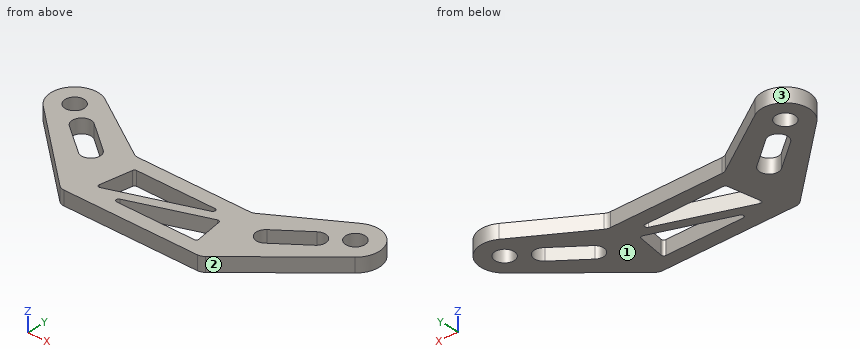
from build123d import *

# Parameters (mm, degrees)
SKETCH_1_R          = 2.025
EXTRUDE_1_DEPTH     = 3
CUT_EXTRUDE_1_DEPTH = 13
FILLET_1_R          = 0.5
FILLET_2_R          = 2


with BuildPart() as part:
    # 草图1 → 凸台-拉伸1 (new body)
    with BuildSketch(Plane.XY):
        with BuildLine():
            Line((-12.5, -5), (-27.339189471, 4.262711851))
            ThreePointArc((-27.339189471, 4.262711851), (-34.026108353, 3.006838294), (-33.33194179, -3.761487592))
            Line((-33.33194179, -3.761487592), (-15, -20))
            Line((-15, -20), (15, -20))
            Line((15, -20), (33.33194179, -3.761487592))
            ThreePointArc((33.33194179, -3.761487592), (34.026108353, 3.006838294), (27.339189471, 4.262711851))
            Line((27.339189471, 4.262711851), (12.5, -5))
            Line((12.5, -5), (-12.5, -5))
        make_face()
        with Locations((-30, 0)):
            Circle(SKETCH_1_R, mode=Mode.SUBTRACT)
        with Locations((30, 0)):
            Circle(SKETCH_1_R, mode=Mode.SUBTRACT)
    extrude(amount=EXTRUDE_1_DEPTH)

    # 草图2 → 切除-拉伸1 (cut)
    with BuildSketch(Plane.XY.offset(3)):
        Polygon((9.958618735, -8), (-9.958618735, -8), (-11.278048465, -15.916578379), align=None)
        Polygon((10.293550357, -10.009589734), (-8.458618735, -17), (11.458618735, -17), align=None)
        with BuildLine():
            Line((17.485082522, -7.103595065), (23.826074435, -2.225908978))
            ThreePointArc((23.826074435, -2.225908978), (26.630743935, -2.591735435), (26.264917478, -5.396404935))
            Line((26.264917478, -5.396404935), (19.923925565, -10.274091022))
            ThreePointArc((19.923925565, -10.274091022), (17.119256065, -9.908264565), (17.485082522, -7.103595065))
        make_face()
        with BuildLine():
            Line((-23.826074435, -2.225908978), (-17.485082522, -7.103595065))
            ThreePointArc((-17.485082522, -7.103595065), (-17.119256065, -9.908264565), (-19.923925565, -10.274091022))
            Line((-19.923925565, -10.274091022), (-26.264917478, -5.396404935))
            ThreePointArc((-26.264917478, -5.396404935), (-26.630743935, -2.591735435), (-23.826074435, -2.225908978))
        make_face()
    extrude(amount=-CUT_EXTRUDE_1_DEPTH, mode=Mode.SUBTRACT)

    # 圆角1
    fillet_1_edges = [part.edges().sort_by_distance(p)[0] for p in [
        (11.458618735, -17, 1.5),
        (-8.458618735, -17, 1.5),
        (10.293550357, -10.009589734, 1.5),
        (-11.278048465, -15.916578379, 1.5),
        (-9.958618735, -8, 1.5),
        (9.958618735, -8, 1.5),
    ]]
    fillet(fillet_1_edges, radius=FILLET_1_R)

    # 圆角2
    fillet_2_edges = [part.edges().sort_by_distance(p)[0] for p in [
        (-12.5, -5, 1.5),
        (12.5, -5, 1.5),
        (15, -20, 1.5),
        (-15, -20, 1.5),
    ]]
    fillet(fillet_2_edges, radius=FILLET_2_R)


solid = part.part
Design review of the part built by this model. Coordinates are the model's own, in mm. Face numbers are marked on the shaded views. Round coordinates to 2 decimals unless told otherwise and drop trailing zeros. Order: outer loops, then holes, each group sorted by start corner. A loop starts at its lowest first (then second) coordinate and runs counter-clockwise, first axis right, second up.
1) Consider section A-A (z = 0.9). Count the separate pieces of the cut face and the enclosed holes in it, plus the area to 3 significant figures.
The answers:
separate pieces: 1
enclosed holes: 6
area: 713 mm2
2) Consider section D-D (x = 30). State the section outline as (y, z) points (3 decimals), plus the area to 3 significant figures.
The answers:
outline: (-6.713, 0) - (-2.025, 0) - (-2.025, 3) - (-6.713, 3) - close; (2.025, 0) - (5.025, 0) - (5.025, 3) - (2.025, 3) - close
area: 23.1 mm2
3) Consider section B-B (x = 8.5). State the section outline as (y, z) points.
The answers:
outline: (-20, 0) - (-17, 0) - (-17, 3) - (-20, 3) - close; (-10.68, 0) - (-5, 0) - (-5, 3) - (-10.68, 3) - close
4) For L1, parallel to X at y = -4.75, z = 1.4; L2, parallel to X at y = -0.75, z = 1.15; L3, parallel to Y at x = -20, z = 2.25, list the stretches that pass through material, from the lowest coordinate up.
The answers:
L1: x = -32.22 to -26.81, -20.54 to -12.9, 12.9 to 20.54, 26.81 to 32.22
L2: x = -34.97 to -31.88, -28.12 to -19.31, 19.31 to 28.12, 31.88 to 34.97
L3: y = -15.57 to -10.22, -5.17 to -0.32
5) Consider section C-C (y = 0). State the section outline as (x, z) points (3 decimals).
The answers:
outline: (-35.025, 0) - (-32.025, 0) - (-32.025, 3) - (-35.025, 3) - close; (-27.975, 0) - (-20.51, 0) - (-20.51, 3) - (-27.975, 3) - close; (20.51, 0) - (27.975, 0) - (27.975, 3) - (20.51, 3) - close; (32.025, 0) - (35.025, 0) - (35.025, 3) - (32.025, 3) - close
6) Clearance check with flat-ended pins moving along their axes: pin 1 Ø0.9 at (x, z) = (2, 1.5) entering from +Y; pin 2 Ø1 at (y, z) = (-15.5, 0.5) entering from +X; pin 3 Ø1.5 at (x, z) = (-14.5, 0.5) entering from +Y. State where each tip first meets the part, or that it passes through.
The answers:
pin 1: stops at y = -5
pin 2: stops at x = 20.64
pin 3: stops at y = -3.28
7) Draft analysis for pull direction X (two halves, no side actions). For the marked faces 1, 2 and 3, state which applies: released by +X, released by -X, zero draft, split by the parting line, or undercut.
The answers:
face 1: zero draft
face 2: released by +X
face 3: undercut
